Check sheet for the modelled part. Datum: model origin and axes. Units: mm. Face numbers are marked on the shaded views. Round coordinates to 2 decimals unless told otherwise and drop trailing zeros. Order: outer loops, then holes, each group sorted by start corner. A loop starts at its lowest first (then second) coordinate and runs counter-clockwise, first axis right, second up.
```python
from build123d import *

# Parameters (mm, degrees)
F0_R     = 12
F0_R_2   = 7.05
F1_DEPTH = 124.5
F2_W     = 3
F2_H     = 24
F3_DEPTH = 2.5


with BuildPart() as f1:
    # F0 (on Front) → F1 (new body)
    with BuildSketch(Plane.XZ):
        with Locations((-12, -12)):
            Circle(F0_R)
        with Locations((-12, -12)):
            Circle(F0_R_2, mode=Mode.SUBTRACT)
    extrude(amount=F1_DEPTH)

    # F2 (on Right) → F3 (cut)
    with BuildSketch(Plane.YZ):
        with Locations((-5.5, -12)):
            Rectangle(F2_W, F2_H)
    extrude(amount=-F3_DEPTH, mode=Mode.SUBTRACT)


solid = f1.part
```
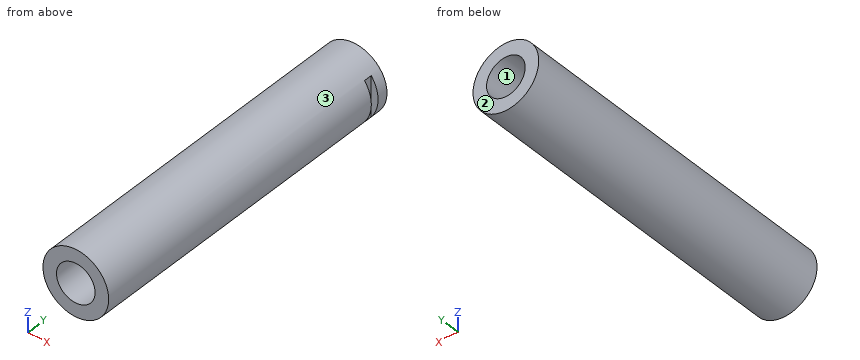
Item 1: Release check for a two-part mould opening along X. For the marked faces 1, 2 and 3 record: released by +X, released by -X, zero draft, split by the parting line, or undercut.
Answer:
face 1: undercut
face 2: zero draft
face 3: split by the parting line
Item 2: Sectioned sample at B-B (z = -12). Record the cut outline in (x, y).
Answer:
outline: (-24, -124.5) - (-19.05, -124.5) - (-19.05, 0) - (-24, 0) - close; (-4.95, -124.5) - (0, -124.5) - (0, -7) - (-2.5, -7) - (-2.5, -4) - (0, -4) - (0, 0) - (-4.95, 0) - close
Item 3: Scan lines: line 1 along Z through (x, y) = (-12, -26.5); line 2 along X through (y, z) = (-105, -8.75); line 3 along X through (y, z) = (-22, -2.5). Record each from-to range of solid material in increasing order.
Answer:
line 1: z = -24 to -19.05, -4.95 to 0
line 2: x = -23.55 to -18.26, -5.74 to -0.45
line 3: x = -19.33 to -4.67
Item 4: Sectioned sample at A-A (x = -12). Record the cut outline in (y, z).
Answer:
outline: (-124.5, -24) - (0, -24) - (0, -19.05) - (-124.5, -19.05) - close; (-124.5, -4.95) - (0, -4.95) - (0, 0) - (-124.5, 0) - close
Item 5: Sectioned sample at D-D (y = -41.5). Record the cut outline in (x, z), and give its area (3 significant figures).
Answer:
outline: circle Ø24 at (-12, -12); hole circle Ø14.1 at (-12, -12)
area: 296 mm2
Item 6: Go/stop test with flat-tipped pins: P1, Ø11.5, axis at x = -12, z = -12, coming from the +Y side; P2, Ø4, axis at x = -5.5, z = -20, coming from the +Y side; P3, Ø1, axis at x = -6, y = -29, coming from the +Z side; P4, Ø4, axis at x = -3.5, y = -91, coming from the +Z side. Record where each tip stops, or that it passes through.
Answer:
P1: passes through
P2: stops at y = 0
P3: stops at z = -1.33
P4: stops at z = -1.91
Item 7: Sectioned sample at C-C (x = -17.75). Record the cut outline in (y, z), and give its area (3 significant figures).
Answer:
outline: (-124.5, -22.53) - (0, -22.53) - (0, -16.08) - (-124.5, -16.08) - close; (-124.5, -7.92) - (0, -7.92) - (0, -1.47) - (-124.5, -1.47) - close
area: 1,610 mm2
